Geometry: final body of the model. Coordinates: model frame, mm. A direction names the side the tool comes from. Give positions to 0.01 mm unless a question says otherwise; leave off trailing zeros. Loops run counter-clockwise (first coordinate to the right, second up) from the corner with the lowest first, then second, coordinate; pieces in that order, holes last. Notation, with made-up numbers: M -11,-8 L 17,-8 A19 cw 17,10 Z; hole C -3.75,49 d3. An arc over 180 degrees is marked long. Put each result on its own line as item: value.
```python
from build123d import *

# Parameters (mm, degrees)
IZIM1_R                     = 0.95
Y_KSEKLIK_EKSTR_ZYON1_DEPTH = 1
RADYUS1_R                   = 0.5
IZIM2_R                     = 1
Y_KSEKLIK_EKSTR_ZYON2_DEPTH = 0.5
RADYUS2_R                   = 0.5
RADYUS3_R                   = 2


with BuildPart() as part:
    # Çizim1 → Yükseklik-Ekstrüzyon1 (new body)
    with BuildSketch(Plane(origin=(0, 0, 0), x_dir=(1, 0, 0), z_dir=(0, 1, 0))):
        with BuildLine():
            Line((-2.5, 5), (-2.5, -5))
            Line((-2.5, -5), (8.506062625, -1.675231512))
            ThreePointArc((8.506062625, -1.675231512), (9.75, 0), (8.506062625, 1.675231512))
            Line((8.506062625, 1.675231512), (-2.5, 5))
        make_face()
        with Locations(Location((0, 2.5, 0), (0, 0, 270))):
            Circle(IZIM1_R, mode=Mode.SUBTRACT)
        with Locations(Location((0, -2.5, 0), (0, 0, 270))):
            Circle(IZIM1_R, mode=Mode.SUBTRACT)
        with Locations(Location((8, 0, 0), (0, 0, 270))):
            Circle(IZIM1_R, mode=Mode.SUBTRACT)
    extrude(amount=Y_KSEKLIK_EKSTR_ZYON1_DEPTH)

    # Radyus1
    radyus1_edges = [part.edges().sort_by_distance(p)[0] for p in [
        (-2.5, 0.5, 5),
        (-2.5, 0.5, -5),
    ]]
    fillet(radyus1_edges, radius=RADYUS1_R)

    # Çizim2 → Yükseklik-Ekstrüzyon2 (add, symmetric)
    with BuildSketch(Plane.XY):
        Polygon((-2.5, 1), (-3.077350269, 2), (-5.6, 2), (-5.6, 14.68320138), (-2.4, 14.68320138), (5.5, 1), align=None)
        with Locations((-4, 4)):
            Circle(IZIM2_R, mode=Mode.SUBTRACT)
        with Locations((-4, 12.68320138)):
            Circle(IZIM2_R, mode=Mode.SUBTRACT)
        with Locations((-4, 8.34160069)):
            Circle(IZIM2_R, mode=Mode.SUBTRACT)
    extrude(amount=Y_KSEKLIK_EKSTR_ZYON2_DEPTH, both=True)

    # Radyus2
    # the kernel refuses this fillet: 0.5 mm, written as the material it adds along each edge
    with BuildSketch(Plane(origin=(6.75, 1, 0.5), x_dir=(0, 0, 1), z_dir=(-1, 0, 0))) as radyus2_piece_1_section:
        with BuildLine():
            CenterArc((RADYUS2_R, RADYUS2_R), RADYUS2_R, 180, 90)
            Line((0, RADYUS2_R), (0, 0))
            Line((0, 0), (RADYUS2_R, 0))
        make_face()
    radyus2_piece_1 = extrude(amount=9.25, mode=Mode.PRIVATE)
    radyus2_piece_1 = split(radyus2_piece_1, bisect_by=Plane(origin=(4.44326915, 2.830311522, 0.613693195), z_dir=(-0.8660254037844398, -0.49999999999999806, 0)), keep=Keep.TOP, mode=Mode.PRIVATE)
    radyus2_piece_1 = split(radyus2_piece_1, bisect_by=Plane(origin=(-1.55673085, -0.633790093, 0.613693195), z_dir=(0.8660254037844397, 0.4999999999999983, 0)), keep=Keep.TOP, mode=Mode.PRIVATE)
    add(radyus2_piece_1)
    with BuildSketch(Plane(origin=(6.75, 1, 0.5), x_dir=(0, 0, 1), z_dir=(-1, 0, 0))) as radyus2_piece_2_section:
        with BuildLine():
            CenterArc((RADYUS2_R, RADYUS2_R), RADYUS2_R, 180, 90)
            Line((0, RADYUS2_R), (0, 0))
            Line((0, 0), (RADYUS2_R, 0))
        make_face()
    radyus2_piece_2 = extrude(amount=10.5, mode=Mode.PRIVATE)
    radyus2_piece_2 = split(radyus2_piece_2, bisect_by=Plane(origin=(-2.5, 1.215059026, 0.553236256), z_dir=(-1, 0, 0)), keep=Keep.TOP, mode=Mode.PRIVATE)
    radyus2_piece_2 = split(radyus2_piece_2, bisect_by=Plane(origin=(-2.608643838, 1.188176648, 0.553236256), z_dir=(0.8660254037844397, 0.4999999999999983, 0)), keep=Keep.TOP, mode=Mode.PRIVATE)
    add(radyus2_piece_2)
    with BuildSketch(Plane(origin=(6.75, 1, -0.5), x_dir=(0, 0, -1), z_dir=(-1, 0, 0))) as radyus2_piece_3_section:
        with BuildLine():
            CenterArc((RADYUS2_R, -RADYUS2_R), RADYUS2_R, 90, 90)
            Line((0, -RADYUS2_R), (0, 0))
            Line((0, 0), (RADYUS2_R, 0))
        make_face()
    radyus2_piece_3 = extrude(amount=9.25, mode=Mode.PRIVATE)
    radyus2_piece_3 = split(radyus2_piece_3, bisect_by=Plane(origin=(4.44326915, 2.830311522, -0.613693195), z_dir=(-0.8660254037844398, -0.49999999999999806, 0)), keep=Keep.TOP, mode=Mode.PRIVATE)
    radyus2_piece_3 = split(radyus2_piece_3, bisect_by=Plane(origin=(-1.55673085, -0.633790093, -0.613693195), z_dir=(0.8660254037844397, 0.4999999999999983, 0)), keep=Keep.TOP, mode=Mode.PRIVATE)
    add(radyus2_piece_3)
    with BuildSketch(Plane(origin=(6.75, 1, -0.5), x_dir=(0, 0, -1), z_dir=(-1, 0, 0))) as radyus2_piece_4_section:
        with BuildLine():
            CenterArc((RADYUS2_R, -RADYUS2_R), RADYUS2_R, 90, 90)
            Line((0, -RADYUS2_R), (0, 0))
            Line((0, 0), (RADYUS2_R, 0))
        make_face()
    radyus2_piece_4 = extrude(amount=10.5, mode=Mode.PRIVATE)
    radyus2_piece_4 = split(radyus2_piece_4, bisect_by=Plane(origin=(-2.5, 1.215059026, -0.553236256), z_dir=(-1, 0, 0)), keep=Keep.TOP, mode=Mode.PRIVATE)
    radyus2_piece_4 = split(radyus2_piece_4, bisect_by=Plane(origin=(-2.608643838, 1.188176648, -0.553236256), z_dir=(0.8660254037844397, 0.4999999999999983, 0)), keep=Keep.TOP, mode=Mode.PRIVATE)
    add(radyus2_piece_4)
    # the kernel refuses this fillet: 0.5 mm, written as the material it takes off along each edge
    with BuildSketch(Plane(origin=(-5.6, 2, 1.75), x_dir=(0, 1, 0), z_dir=(0, 0, -1))) as radyus2_2_piece_1:
        with BuildLine():
            CenterArc((RADYUS2_R, RADYUS2_R), RADYUS2_R, 180, 90)
            Line((0, RADYUS2_R), (0, 0))
            Line((0, 0), (RADYUS2_R, 0))
        make_face()
    extrude(amount=3.5, mode=Mode.SUBTRACT)

    # Radyus3
    radyus3_edges = [part.edges().sort_by_distance(p)[0] for p in [
        (-5.6, 14.68320138, 0),
        (-2.4, 14.68320138, 0),
    ]]
    fillet(radyus3_edges, radius=RADYUS3_R)


solid = part.part
```
Item 1: Set-up query: faces 5 (the flat face through (-1, 7, -0.5)), 6 (the flat face through (-1, 7, 0.5)), 7 (the flat face through (-4, 2, 0)). Return all of +Z, -Z, +X, -X, +Y, -Y with unobstructed straight access to the full face (end or side cutting, diameter ignored); none if empty.
Output values:
face 5: -Z, +X, -X, +Y
face 6: +Z, +X, -X, +Y
face 7: +Z, -Z, -X, -Y
Item 2: Section D-D on z = -2.5. Output: boundary loops of the cut face in (x, y), then the cut area to 3 significant figures.
Output values:
outline: M -2.5,0 L -0.95,0 L -0.95,1 L -2.5,1 Z; M 0.95,0 L 5.78,0 L 5.78,1 L 0.95,1 Z
area: 6.38 mm²
Item 3: Line query: probe 1 along Y at (x, z) = (-4, 0.1); probe 2 along Y at (x, z) = (1, 3); probe 3 along Z at (x, y) = (-1, 2.25). Output: solid intervals per line, ascending. Write a range as [from, to].
Output values:
probe 1: [2, 3], [5, 7.34], [9.34, 11.68], [13.68, 14.64]
probe 2: [0, 1]
probe 3: [-0.5, 0.5]
Item 4: Mould query, pull axis X, two halves, no side actions, for faces 1 (the flat face through (2, 0, 0)), 2 (the cylindrical face through (-4.79, 12.07, -0.01)), 3 (the flat face through (-2.5, 0.5, -0.1)), 4 (the cylindrical face through (0.04, 0.49, -3.45)). Classes: pulls with the +X half, pulls with the -X half, needs draft (parallel to the pull), parting line crosses it, or undercut.
Output values:
face 1: needs draft
face 2: undercut
face 3: pulls with the -X half
face 4: undercut
Item 5: Pin query (flat end, axial travel): pin 1 Ø8.5 at (x, y) = (-1.5, 8) entering from -Z; pin 2 Ø3 at (x, z) = (0, 2.5) entering from +Y; pin 3 Ø5 at (x, y) = (5.5, 7) entering from -Z; pin 4 Ø6 at (x, y) = (4.5, 1.5) entering from -Z. Return the tip coordinate at first contact, or that it passes through.
Output values:
pin 1: z = -0.5
pin 2: y = 1
pin 3: through
pin 4: z = -3.78
Item 6: Section C-C on x = 0.25. Output: boundary loops of the cut face in (y, z), then the cut area to 3 significant figures.
Output values:
outline: M 0,-4.17 L 1,-4.17 L 1,-3.42 L 0,-3.42 Z; M 0,-1.58 L 1,-1.58 L 1,-1 A0.5 cw 1.5,-0.5 L 10.09,-0.5 L 10.09,0.5 L 1.5,0.5 A0.5 cw 1,1 L 1,1.58 L 0,1.58 Z; M 0,3.42 L 1,3.42 L 1,4.17 L 0,4.17 Z
area: 13.9 mm²
Item 7: Section A-A on z = 0. Output: boundary loops of the cut face in (x, y).
Output values:
outline: M -5.6,2.5 A0.5 ccw -5.1,2 L -3.08,2 L -2.5,1 L -2.5,0 L 7.05,0 L 7.05,1 L 5.5,1 L -1.82,13.68 A2 ccw -3.55,14.68 L -3.6,14.68 A2 ccw -5.6,12.68 Z; M 8.95,0 L 9.75,0 L 9.75,1 L 8.95,1 Z; hole C -4,4 d2; hole C -4,8.34 d2; hole C -4,12.68 d2
Item 8: Section B-B on y = 4. Output: boundary loops of the cut face in (x, z).
Output values:
outline: M -5.6,-0.5 L -5,-0.5 L -5,0.5 L -5.6,0.5 Z; M -3,-0.5 L 3.77,-0.5 L 3.77,0.5 L -3,0.5 Z
